The model under review builds one solid part; all positions refer to its coordinate system, in mm. Face numbers are marked on the shaded views. A direction names the side the tool comes from. Coordinates: 2 decimals unless noted, no trailing zeros. Write each loop counter-clockwise with the first axis right and the second up, starting at its lowest first coordinate (ties: lowest second). Pieces come first, ordered by that corner, then holes.
```python
from build123d import *

# Parameters (mm, degrees)
CROQUIS1_W              = 300
CROQUIS1_H              = 195
SALIENTE_EXTRUIR1_DEPTH = 16
CROQUIS2_W              = 16
CROQUIS2_H              = 195
SALIENTE_EXTRUIR2_DEPTH = 220
CROQUIS7_W              = 300
CROQUIS7_H              = 195
SALIENTE_EXTRUIR4_DEPTH = 16
CROQUIS8_W              = 268
CROQUIS8_H              = 128
SALIENTE_EXTRUIR5_DEPTH = 16
CROQUIS11_W             = 41
CROQUIS11_H             = 35
SALIENTE_EXTRUIR6_DEPTH = 20


with BuildPart() as part:
    # Croquis1 → Saliente-Extruir1 (new body)
    with BuildSketch(Plane(origin=(0, 0, 0), x_dir=(1, 0, 0), z_dir=(0, 1, 0))):
        Rectangle(CROQUIS1_W, CROQUIS1_H)
    extrude(amount=SALIENTE_EXTRUIR1_DEPTH)

    # Croquis2 → Saliente-Extruir2 (add)
    with BuildSketch(Plane(origin=(0, 16, 0), x_dir=(1, 0, 0), z_dir=(0, 1, 0))):
        with Locations((-142, 0)):
            Rectangle(CROQUIS2_W, CROQUIS2_H)
        with Locations((142, 0)):
            Rectangle(CROQUIS2_W, CROQUIS2_H)
    extrude(amount=SALIENTE_EXTRUIR2_DEPTH)

    # Croquis7 → Saliente-Extruir4 (add)
    with BuildSketch(Plane(origin=(0, 236, 0), x_dir=(1, 0, 0), z_dir=(0, 1, 0))):
        Rectangle(CROQUIS7_W, CROQUIS7_H)
    extrude(amount=SALIENTE_EXTRUIR4_DEPTH)

    # Croquis8 → Saliente-Extruir5 (add)
    with BuildSketch(Plane(origin=(0, 94.5, 0), x_dir=(1, 0, 0), z_dir=(0, 1, 0))):
        with Locations((0, 33.5)):
            Rectangle(CROQUIS8_W, CROQUIS8_H)
    extrude(amount=SALIENTE_EXTRUIR5_DEPTH)

    # Croquis11 → Saliente-Extruir6 (add)
    with BuildSketch(Plane(origin=(0, 110.5, 0), x_dir=(1, 0, 0), z_dir=(0, 1, 0))):
        with Locations((10.868818232, 64.486978539)):
            Rectangle(CROQUIS11_W, CROQUIS11_H)
    extrude(amount=SALIENTE_EXTRUIR6_DEPTH)


solid = part.part
```
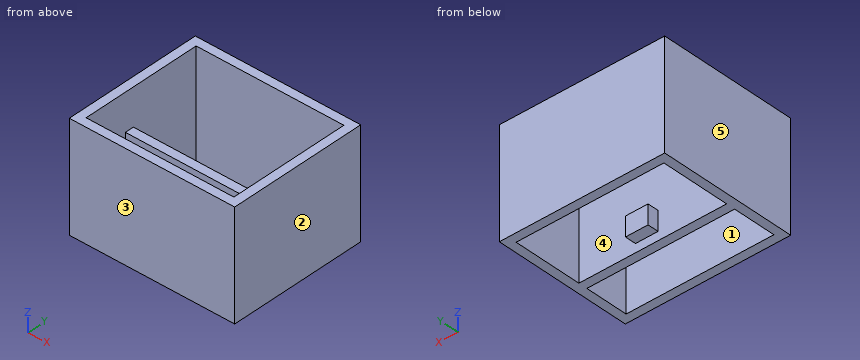
Item 1: Take a section at C-C, the plane z = 9.5. Write out the cut boundary in (x, y), plus the area to 3 significant figures.
Solved:
outline: (-150, 0) - (150, 0) - (150, 252) - (-150, 252) - close; hole (-134, 16) - (134, 16) - (134, 94.5) - (-134, 94.5) - close; hole (-134, 110.5) - (134, 110.5) - (134, 236) - (-134, 236) - close
area: 20,900 mm2
Item 2: Machinability: for the marked faces 1 and 2, which of the approach directions +Z, -Z, +X, -X, +Y, -Y give a long, thin tool a straight path to every point of the face, cutting with its end or side? Answer none if there is none.
Solved:
face 1: +Z, -Z
face 2: +Z, -Z, +X, +Y, -Y
Item 3: Take a section at A-A, the plane y = 219.5. Write out the cut boundary in (x, z).
Solved:
outline: (-150, -97.5) - (-134, -97.5) - (-134, 97.5) - (-150, 97.5) - close; (134, -97.5) - (150, -97.5) - (150, 97.5) - (134, 97.5) - close
Item 4: For pin 1 (6 mm diameter, centred on x = 18, y = 122.5, fed in from -Z); pin 2 (2 mm diameter, centred on x = 82.5, z = 33, fed in from -Y); pin 3 (10 mm diameter, centred on x = 3, y = 118.5, fed in from +Z); pin 4 (5 mm diameter, centred on x = -3, y = 104, fed in from +Z), all flat-tipped, find the tip position at first contact; note any pin that passes through.
Solved:
pin 1: stops at z = -81.99
pin 2: stops at y = 0
pin 3: stops at z = -46.99
pin 4: stops at z = 30.5
Item 5: Take a section at B-B, the plane x = 12.5. Write out the cut boundary in (y, z), plus the area to 3 significant figures.
Solved:
outline: (0, -97.5) - (16, -97.5) - (16, 97.5) - (0, 97.5) - close; (94.5, -97.5) - (110.5, -97.5) - (110.5, -81.99) - (130.5, -81.99) - (130.5, -46.99) - (110.5, -46.99) - (110.5, 30.5) - (94.5, 30.5) - close; (236, -97.5) - (252, -97.5) - (252, 97.5) - (236, 97.5) - close
area: 8,990 mm2
Item 6: Mouldability with a two-part tool opening along Y and no side actions: class the marked faces 3, 4 and 5 as pulls with the +Y half, pulls with the -Y half, needs draft (parallel to the pull), parting line crosses it, or undercut.
Solved:
face 3: pulls with the -Y half
face 4: undercut
face 5: needs draft
Item 7: To check wall thickness, follow line 1 along Y through (x, z) = (133, -50.5); line 2 along X through (y, z) = (166, 86.5); line 3 along Y through (x, z) = (-6.5, 78). State the ranges of each line that lie inside material, in increasing order.
Solved:
line 1: y = 0 to 16, 94.5 to 110.5, 236 to 252
line 2: x = -150 to -134, 134 to 150
line 3: y = 0 to 16, 236 to 252
Item 8: Take a section at D-D, the plane y = 120.5. Write out the cut boundary in (x, z), plus the area to 4 significant figures.
Solved:
outline: (-150, -97.5) - (-134, -97.5) - (-134, 97.5) - (-150, 97.5) - close; (-9.63, -81.99) - (31.37, -81.99) - (31.37, -46.99) - (-9.63, -46.99) - close; (134, -97.5) - (150, -97.5) - (150, 97.5) - (134, 97.5) - close
area: 7,675 mm2
